```python
from build123d import *

# Parameters (mm, degrees)
F1_DEPTH = 50.8
F3_R     = 5.08


# Not quite as in the source:
# - the program builds the solid bodies; features that only make, move or delete a surface that nothing else refers to are left out


with BuildPart() as f1:
    # F0 (on Front) → F1 (new body)
    with BuildSketch(Plane.XZ):
        with BuildLine():
            Line((25.4, 0), (12.7, 0))
            ThreePointArc((12.7, 0), (-8.9802561211, -8.9802561211), (0, 12.7))
            Line((0, 12.7), (0, 25.4))
            Line((0, 25.4), (-25.4, 25.4))
            Line((-25.4, 25.4), (-25.4, 0))
            Line((-25.4, 0), (-25.4, -25.4))
            Line((-25.4, -25.4), (0, -25.4))
            Line((0, -25.4), (25.4, -25.4))
            Line((25.4, -25.4), (25.4, 0))
        make_face()
        with BuildLine():
            ThreePointArc((0, 12.7), (8.9802561211, 8.9802561211), (12.7, 0))
            Line((12.7, 0), (25.4, 0))
            Line((25.4, 0), (25.4, 25.4))
            Line((25.4, 25.4), (0, 25.4))
            Line((0, 25.4), (0, 12.7))
        make_face()
    extrude(amount=F1_DEPTH)

    # F3
    f3_edges = [f1.edges().sort_by_distance(p)[0] for p in [
        (-25.4, -25.4, 25.4),
        (25.4, -25.4, 25.4),
        (-25.4, -25.4, -25.4),
        (25.4, -25.4, -25.4),
        (25.4, 0, 0),
        (-25.4, 0, 0),
        (-25.4, -50.8, 0),
        (25.4, -50.8, 0),
    ]]
    fillet(f3_edges, radius=F3_R)


solid = f1.part
```
Verification items for the finished model (mm, model axes). Round coordinates to 2 decimals unless told otherwise and drop trailing zeros. Write each loop counter-clockwise with the first axis right and the second up, starting at its lowest first coordinate (ties: lowest second). Pieces come first, ordered by that corner, then holes. Notation, with made-up numbers: (-8.75, 69.5) -> (43.25, 69.5) arc R18 cw to (43.25, 73.5) -> close; hole circle Ø10 at (77.25, 85). An arc over 180 degrees is marked (long way). Write each question's results on one line, items separated by ' | '. Start each with the question number.
1. Cross-section at C-C (z = 1). Enter the section's corners in (x, y).
2. Cross-section at B-B (x = -8). Enter the section's corners in (y, z), then the cut area to 3 significant figures.
3. Cross-section at D-D (x = 5). Enter the section's corners in (y, z).
4. Cross-section at A-A (y = -6.5). Enter the section's corners in (x, z).
5. Material ranges on probe 1 along Z at (x, y) = (0, -22.5); probe 2 along X at (y, z) = (-21, -3), recorded low to high. Write a range as from..to.
Solutions:
1) outline: (-25.4, -45.72) arc R5.08 ccw to (-20.32, -50.8) -> (-12.66, -50.8) -> (-12.66, 0) -> (-20.32, 0) arc R5.08 ccw to (-25.4, -5.08) -> close; (12.66, -50.8) -> (20.32, -50.8) arc R5.08 ccw to (25.4, -45.72) -> (25.4, -5.08) arc R5.08 ccw to (20.32, 0) -> (12.66, 0) -> close
2) outline: (-50.8, -25.4) -> (0, -25.4) -> (0, -9.86) -> (-50.8, -9.86) -> close; (-50.8, 9.86) -> (0, 9.86) -> (0, 25.4) -> (-50.8, 25.4) -> close | area: 1,580 mm2
3) outline: (-50.8, -25.4) -> (0, -25.4) -> (0, -11.67) -> (-50.8, -11.67) -> close; (-50.8, 11.67) -> (0, 11.67) -> (0, 25.4) -> (-50.8, 25.4) -> close
4) outline: (-25.4, -20.32) arc R5.08 ccw to (-20.32, -25.4) -> (20.32, -25.4) arc R5.08 ccw to (25.4, -20.32) -> (25.4, 20.32) arc R5.08 ccw to (20.32, 25.4) -> (-20.32, 25.4) arc R5.08 ccw to (-25.4, 20.32) -> close; hole circle Ø25.4 at (0, 0)
5) probe 1: z = -25.4..-12.7, 12.7..25.4 | probe 2: x = -25.4..-12.34, 12.34..25.4
